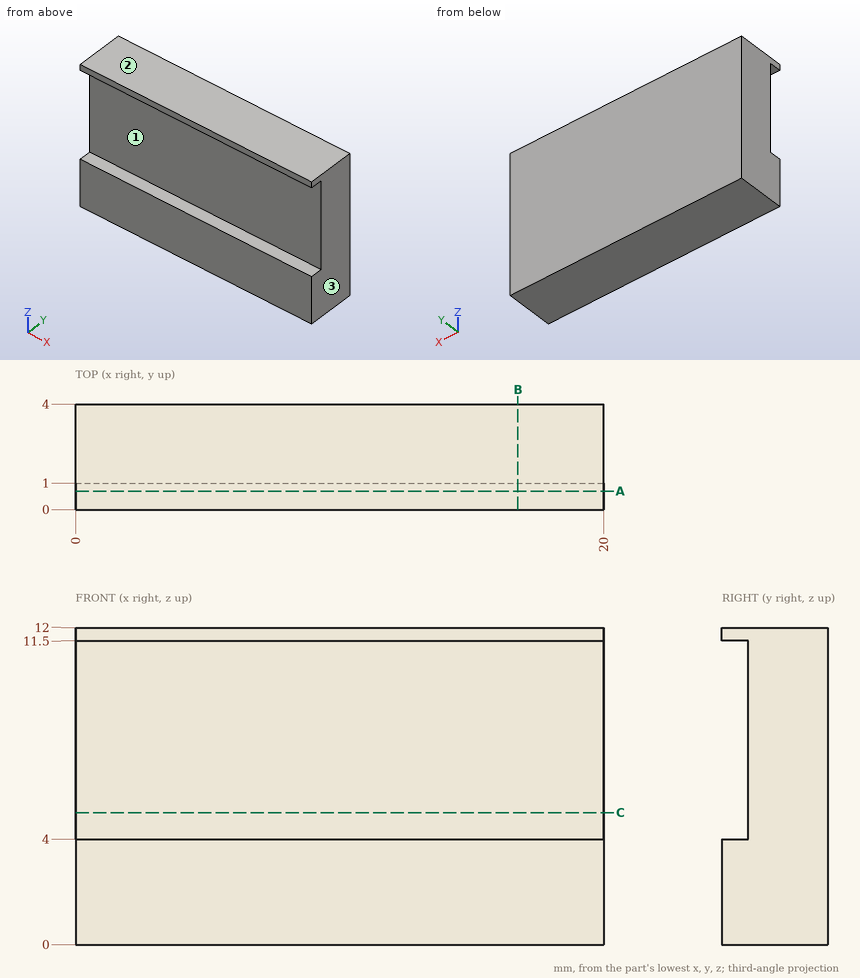
Verification items for this drawing (mm, ordinates from the low corner). Coordinates: 2 decimals unless noted, no trailing zeros. Write each loop counter-clockwise with the first axis right and the second up, starting at its lowest first coordinate (ties: lowest second). Pieces come first, ordered by that corner, then holes. Notation, with made-up numbers: M 42.5,-22.5 L 71.5,-22.5 A15 ccw 71.5,1.5 Z; hole C 55,54 d4. An arc over 180 degrees is marked long. One line per item, written item: value. Start each with the question number.
(1) Sectioned sample at B-B, the plane x = 16.75. Enter the section's corners in (y, z), and give its area (3 significant figures).
(2) Release check for a two-part mould opening along Z. For the marked faces 1, 2 and 3 record: released by +Z, released by -Z, zero draft, split by the parting line, or undercut.
(3) Sectioned sample at C-C, the plane z = 5. Enter the section's corners in (x, y).
(4) Scan lines: line 1 along Z through (x, y) = (12.75, 0.4); line 2 along Y through (x, z) = (13, 8.75). Record each from-to range of solid material in increasing order. Write a range as [from, to].
(5) Sectioned sample at A-A, the plane y = 0.7. Enter the section's corners in (x, z), and give its area (3 significant figures).
Filled sheet:
1. outline: M 0,0 L 4,0 L 4,12 L 0,12 L 0,11.5 L 1,11.5 L 1,4 L 0,4 Z
1. area: 40.5 mm²
2. face 1: undercut
2. face 2: released by +Z
2. face 3: zero draft
3. outline: M 0,1 L 20,1 L 20,4 L 0,4 Z
4. line 1: [0, 4], [11.5, 12]
4. line 2: [1, 4]
5. outline: M 0,0 L 20,0 L 20,4 L 0,4 Z; M 0,11.5 L 20,11.5 L 20,12 L 0,12 Z
5. area: 90.0 mm²
